```python
from build123d import *

# Parameters (mm, degrees)
SKETCH1_R           = 4
BOSS_EXTRUDE1_DEPTH = 6
FILLET1_R           = 1


with BuildPart() as part:
    # Sketch1 → Boss-Extrude1 (new body)
    with BuildSketch(Plane(origin=(0, 0, 0), x_dir=(1, 0, 0), z_dir=(0, 1, 0))):
        Polygon((7.505553499, 0), (3.75277675, 6.5), (-3.75277675, 6.5), (-7.505553499, 0), (-3.75277675, -6.5), (3.75277675, -6.5), align=None)
        Circle(SKETCH1_R, mode=Mode.SUBTRACT)
    extrude(amount=BOSS_EXTRUDE1_DEPTH)

    # Fillet1
    fillet1_edges = [part.edges().sort_by_distance(p)[0] for p in [
        (0, 6, -6.5),
        (-5.629165125, 6, -3.25),
        (-5.629165125, 6, 3.25),
        (0, 6, 6.5),
        (5.629165125, 6, 3.25),
        (0, 0, 6.5),
        (-5.629165125, 0, 3.25),
        (-5.629165125, 0, -3.25),
        (0, 0, -6.5),
        (5.629165125, 0, -3.25),
        (5.629165125, 0, 3.25),
        (5.629165125, 6, -3.25),
    ]]
    fillet(fillet1_edges, radius=FILLET1_R)


solid = part.part
```
Source: CAD feature listing. Evaluate the final solid. Frame: model axes, mm. Round coordinates to 2 decimals unless told otherwise and drop trailing zeros. Loops run counter-clockwise (first coordinate to the right, second up) from the corner with the lowest first, then second, coordinate; pieces in that order, holes last. Notation, with made-up numbers: M 25,-8.5 L 36,-8.5 A29 ccw 36,22.5 Z; hole C 30.5,-22 d9. An arc over 180 degrees is marked long. Use a Markdown table: item, result. Add a question column.
1. Cut plane B-B, the plane x = 0. Output: boundary loops of the cut face in (y, z), and give its area (3 significant figures).
2. Cut plane A-A, the plane y = 2.8. Output: boundary loops of the cut face in (x, z).
3. Ray query, line 1 along Z through (x, y) = (0, 1.5); line 2 along X through (y, z) = (2.75, 0.5); line 3 along X through (y, z) = (3.95, -2.25). Return the intervals inside material, ascending. Write a range as [from, to].
4. Cut plane C-C, the plane y = 5.2. Output: boundary loops of the cut face in (x, z).
5. Pull-direction query (X, two-part tool) for faces 1 (the cylindrical face through (-0.867, 2.958, 3.905)), 2 (the flat face through (0, 3, -6.5)), 3 (the cylindrical face through (-5.41, 0.3, -3.06)); classes: +X half, -X half, draft (parallel to the pull), parting line (faces both ways), or undercut.
6. Contact query for flat-ended pins moving along their axis: pin 1 (3 mm diameter, centred on y = 4, z = -3, fed in from +X); pin 2 (2 mm diameter, centred on y = 1.5, z = 2, fed in from +X). Output: stop coordinate, or through.
Solution:
| question | item | result |
|---|---|---|
| 1 | outline | M 0,-5.5 A1 ccw 1,-6.5 L 5,-6.5 A1 ccw 6,-5.5 L 6,-4 L 0,-4 Z; M 0,4 L 6,4 L 6,5.5 A1 ccw 5,6.5 L 1,6.5 A1 ccw 0,5.5 Z |
| 1 | area | 29.1 mm2 |
| 2 | outline | M -7.51,0 L -3.75,-6.5 L 3.75,-6.5 L 7.51,0 L 3.75,6.5 L -3.75,6.5 Z; hole C 0,0 d8 |
| 3 | line 1 | z = [-6.5, -4], [4, 6.5] |
| 3 | line 2 | x = [-7.22, -3.97], [3.97, 7.22] |
| 3 | line 3 | x = [-6.21, -3.31], [3.31, 6.21] |
| 4 | outline | M -7.48,0 L -3.74,-6.48 L 3.74,-6.48 L 7.48,0 L 3.74,6.48 L -3.74,6.48 Z; hole C 0,0 d8 |
| 5 | face 1 | undercut |
| 5 | face 2 | draft |
| 5 | face 3 | -X half |
| 6 | pin 1 | stops at x = 6.64 |
| 6 | pin 2 | stops at x = 6.93 |
